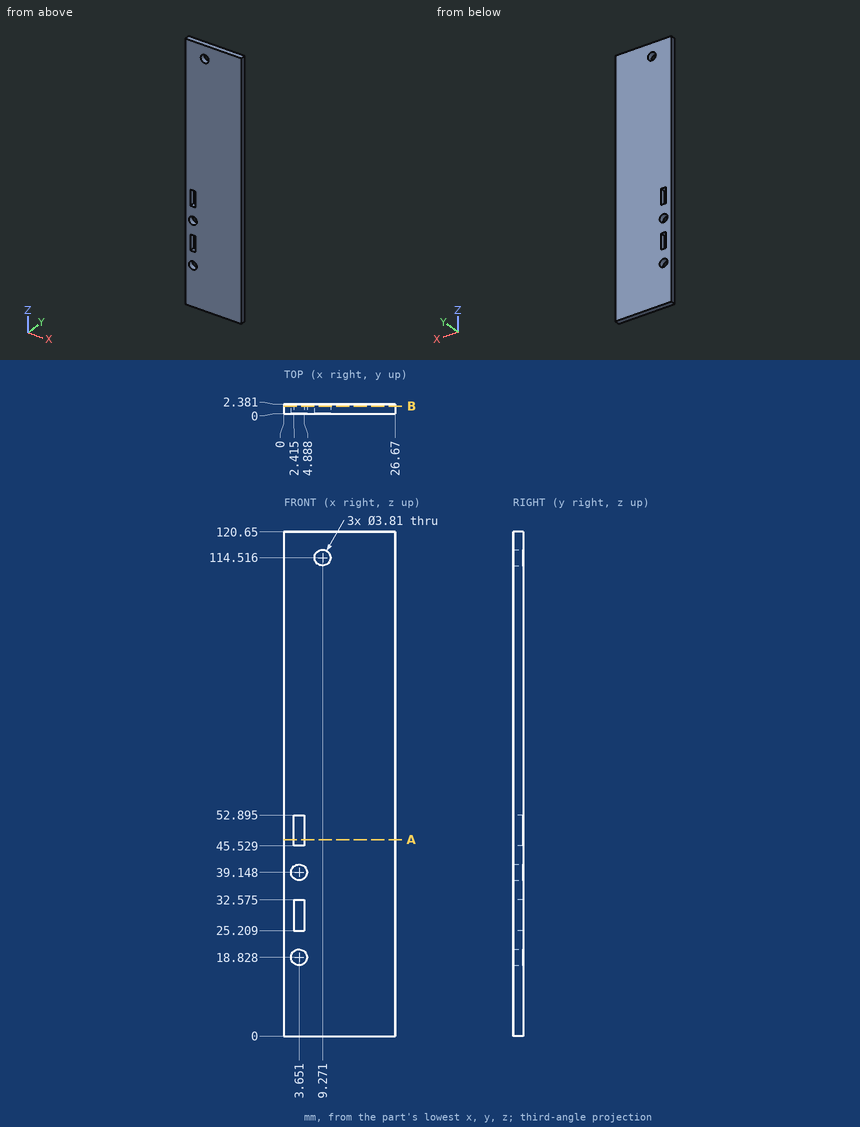
Geometry: see drawing. Coordinates: mm, zero at the bounding-box minimum. Round coordinates to 2 decimals unless told otherwise and drop trailing zeros. Write each loop counter-clockwise with the first axis right and the second up, starting at its lowest first coordinate (ties: lowest second). Pieces come first, ordered by that corner, then holes. Notation, with made-up numbers: (77.25, 13) - (133.25, 13) arc R19 cw to (133.25, 23) - close; hole circle Ø10 at (-5, 32). An arc over 180 degrees is marked (long way). Use CSV: the item, a comma, the result in double quotes. Start each with the question number.
(1) Material intervals for probe 1 along X at (y, z) = (2.25, 52) (1 decimal); probe 2 along Z at (x, y) = (10.25, 2.25); probe 3 along X at (y, z) = (1.65, 114.5) (1 decimal), sorted ascending. Write a range as [from, to].
(2) Cut plane A-A, the plane z = 47. Return loops of the section in (x, y) (1 decimal).
(3) Cut plane B-B, the plane y = 1.85. Give the number of separate pieces and of enclosed holes in the cut face, and give its area (3 significant figures).
Geometry says:
1,probe 1,"[0, 2.4], [4.9, 26.7]"
1,probe 2,"[0, 112.88], [116.15, 120.65]"
1,probe 3,"[0, 7.4], [11.2, 26.7]"
2,outline,"(0, 0) - (2.4, 0) - (2.4, 2.4) - (0, 2.4) - close; (4.9, 0) - (26.7, 0) - (26.7, 2.4) - (4.9, 2.4) - close"
3,separate pieces,"1"
3,enclosed holes,"5"
3,area,"3,150 mm²"
